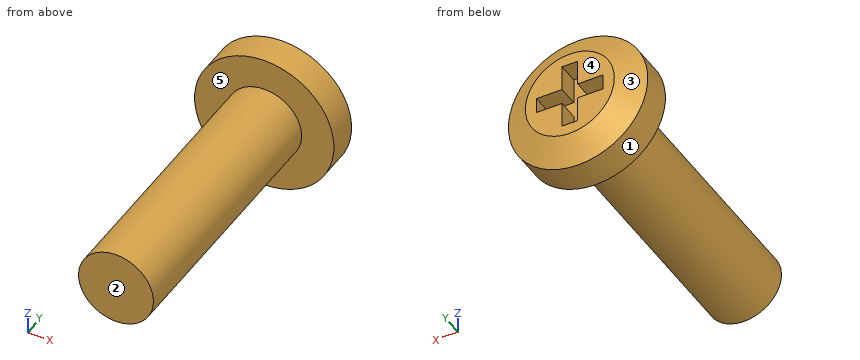
from build123d import *

# Parameters (mm, degrees)
SKETCH1_R           = 3.35
BOSS_EXTRUDE1_DEPTH = 1.5
SKETCH2_R           = 3.35
BOSS_EXTRUDE2_DEPTH = 0.7
BOSS_EXTRUDE2_TAPER = 60
SKETCH3_W           = 1.225
SKETCH3_H           = 0.75
SKETCH3_W_2         = 0.75
SKETCH3_H_2         = 1.225
CUT_EXTRUDE1_DEPTH  = 1
SKETCH4_R           = 1.8
BOSS_EXTRUDE3_DEPTH = 12.6


with BuildPart() as part:
    # Sketch1 → Boss-Extrude1 (new body)
    with BuildSketch(Plane(origin=(0, 0, 0), x_dir=(1, 0, 0), z_dir=(0, 1, 0))):
        with Locations(Location((0, 0, 0), (0, 0, 270))):
            Circle(SKETCH1_R)
    extrude(amount=BOSS_EXTRUDE1_DEPTH)

    # Sketch2 → Boss-Extrude2 (add)
    with BuildSketch(Plane(origin=(0, 1.5, 0), x_dir=(1, 0, 0), z_dir=(0, 1, 0))):
        with Locations(Location((0, 0, 0), (0, 0, 270))):
            Circle(SKETCH2_R)
    extrude(amount=BOSS_EXTRUDE2_DEPTH, taper=BOSS_EXTRUDE2_TAPER)

    # Sketch3 → Cut-Extrude1 (cut)
    with BuildSketch(Plane(origin=(0, 2.2, 0), x_dir=(1, 0, 0), z_dir=(0, 1, 0))):
        with Locations((-0.9875, 0)):
            Rectangle(SKETCH3_W, SKETCH3_H)
        with Locations((0, 0.9875)):
            Rectangle(SKETCH3_W_2, SKETCH3_H_2)
        with Locations((0.9875, 0)):
            Rectangle(SKETCH3_W, SKETCH3_H)
        with Locations((0, -0.9875)):
            Rectangle(SKETCH3_W_2, SKETCH3_H_2)
        Rectangle(SKETCH3_W_2, SKETCH3_H)
    extrude(amount=-CUT_EXTRUDE1_DEPTH, mode=Mode.SUBTRACT)

    # Sketch4 → Boss-Extrude3 (add)
    with BuildSketch(Plane.XZ):
        with Locations(Location((0, 0, 0), (0, 0, 90))):
            Circle(SKETCH4_R)
    extrude(amount=BOSS_EXTRUDE3_DEPTH)


solid = part.part
Could you check a few things on this model? Use its own coordinates, in mm. Face numbers are marked on the shaded views. A direction names the side the tool comes from. Give positions to 0.01 mm unless a question says otherwise; leave off trailing zeros. Order: outer loops, then holes, each group sorted by start corner. A loop starts at its lowest first (then second) coordinate and runs counter-clockwise, first axis right, second up. Notation, with made-up numbers: (81, -35.75) - (127, -35.75) arc R14 ccw to (127, -28.75) - close; hole circle Ø7 at (-27.5, 64.5). An arc over 180 degrees is marked (long way). One line per question, with ' | ' between items. Start each with the question number.
Item 1: I'm going to push flat-ended pins straight in: pin 1 Ø0.5 at (y, z) = (1.5, -1) entering from +X; pin 2 Ø3 at (x, y) = (-1.5, -5.5) entering from +Z; pin 3 Ø0.5 at (y, z) = (2, 1) entering from -X. Where does each tip first touch, or does it pass through?
Item 2: I want a section at A-A on z = 0. Write out the boundary of the cut face in (x, y), then the cut area to 3 significant figures.
Item 3: I want a section at B-B on y = 1. Write out the boundary of the cut face in (x, z).
Item 4: Thinking about a two-plate mould opening in Y: for the marked faces 1, 2 and 3, which applies, pulls with the +Y half, pulls with the -Y half, needs draft (parallel to the pull), parting line crosses it, or undercut?
Item 5: I need wall thicknesses on probe 1 along Y at (x, z) = (-1, -0.25); probe 2 along Z at (x, y) = (1.5, -5.25); probe 3 along Z at (x, y) = (-0.75, -6). Which ranges of each line are inside material? Lowest first, please. Write a range as [from, to].
Item 6: For the marked faces 4 and 5, which set-ups out of +Z, -Z, +X, -X, +Y, -Y let a thin tool reach every point of the face, with its end or its side?
Item 7: I want a section at C-C on y = -4.5. Write out the boundary of the cut face in (x, z), then the cut area to 3 significant figures.
Verdict:
1) pin 1: x = 3.26 | pin 2: z = 1.8 | pin 3: x = -2.75
2) outline: (-3.35, 0) - (-1.8, 0) - (-1.8, -12.6) - (1.8, -12.6) - (1.8, 0) - (3.35, 0) - (3.35, 1.5) - (2.14, 2.2) - (1.6, 2.2) - (1.6, 1.2) - (-1.6, 1.2) - (-1.6, 2.2) - (-2.14, 2.2) - (-3.35, 1.5) - close | area: 56.1 mm^2
3) outline: circle Ø6.7 at (0, 0)
4) face 1: needs draft | face 2: pulls with the -Y half | face 3: pulls with the +Y half
5) probe 1: [-12.6, 1.2] | probe 2: [-0.99, 0.99] | probe 3: [-1.64, 1.64]
6) face 4: +Z, -Z, +X, -X, +Y | face 5: -Y
7) outline: circle Ø3.6 at (0, 0) | area: 10.2 mm^2
